```python
from build123d import *

# Parameters (mm, degrees)
F0_W           = 38.1
F0_H           = 6.35
F1_DEPTH       = 254
F3_D           = 9
F4_D           = 6
F4_CBORE_D     = 11
F4_CBORE_DEPTH = 3


with BuildPart() as f1:
    # F0 (on Top) → F1 (new body)
    with BuildSketch(Plane.XY):
        with Locations((19.05, 3.175)):
            Rectangle(F0_W, F0_H)
    extrude(amount=F1_DEPTH)

    # F3 (through all)
    with Locations(Plane.XZ):
        with Locations((19.05, 25.4), (19.05, 228.6)):
            Hole(F3_D / 2)

    # F4 (through all)
    with Locations(Plane.XZ):
        with Locations((19.05, 172.0088), (19.05, 81.9912)):
            CounterBoreHole(F4_D / 2, F4_CBORE_D / 2, F4_CBORE_DEPTH)


solid = f1.part
```
The listing builds one solid part. Answer for the finished solid, in the listing's coordinates (mm). A direction names the side the tool comes from. Coordinates: 2 decimals unless noted, no trailing zeros. Order: outer loops, then holes, each group sorted by start corner. A loop starts at its lowest first (then second) coordinate and runs counter-clockwise, first axis right, second up. Notation, with made-up numbers: M 38,34 L 87,34 A19 ccw 87,53 Z; hole C 19.5,-13 d10. An arc over 180 degrees is marked long. Answer as a JSON object with one key per item and string values. Group by question number.
1. Straight lines are drawn through the part: line 1 (Z direction, x = 19.05, y = 5); line 2 (Z direction, x = 19.05, y = 1.15); line 3 (X direction, y = 6.25, z = 82.5). For each, find the intervals that lie inside material, in ascending order.
2. A tool of negligible diameter and unlimited length cuts with its end or side. For faces 4 (the flat face through (21.4, 3, 169.6)), 5 (the cylindrical face through (20, 3, 233)), from which of +Z, -Z, +X, -X, +Y, -Y can it reach the whole face along a straight path? Write none if from no direction.
3. Section B-B on z = 228.6 is taken. Write down the section's boundary in (x, y).
4. Flat-ended cylindrical pins translate along their axes: P1, Ø10.5, axis at x = 19.05, z = 228.6, coming from the +Y side; P2, Ø7, axis at x = 19.05, z = 81.99, coming from the -Y side. Find the tip coordinate at first contact, or state that the pin passes through.
5. Section A-A on x = 19.05 is taken. Write down the section's boundary in (y, z), then the cut area to 3 significant figures.
6. Determine the mould class of faces 1 (the cylindrical face through (18.33, 1.48, 177.46)), 2 (the flat face through (0, 3, 125)), 3 (the flat face through (19, 0, 125)) for opening direction X: released by +X, released by -X, zero draft, split by the parting line, or undercut.
7. Section C-C on y = 2 is taken. Write down the section's boundary in (x, z).
Values follow:
{
 "1": {"line 1": "0 to 20.9, 29.9 to 78.99, 84.99 to 169.01, 175.01 to 224.1, 233.1 to 254", "line 2": "0 to 20.9, 29.9 to 76.49, 87.49 to 166.51, 177.51 to 224.1, 233.1 to 254", "line 3": "0 to 16.09, 22.01 to 38.1"},
 "2": {"face 4": "-Y", "face 5": "+Y, -Y"},
 "3": {"outline": "M 0,0 L 14.55,0 L 14.55,6.35 L 0,6.35 Z; M 23.55,0 L 38.1,0 L 38.1,6.35 L 23.55,6.35 Z"},
 "4": {"P1": "y = 6.35", "P2": "y = 3"},
 "5": {"outline": "M 0,0 L 6.35,0 L 6.35,20.9 L 0,20.9 Z; M 0,29.9 L 6.35,29.9 L 6.35,78.99 L 3,78.99 L 3,76.49 L 0,76.49 Z; M 0,87.49 L 3,87.49 L 3,84.99 L 6.35,84.99 L 6.35,169.01 L 3,169.01 L 3,166.51 L 0,166.51 Z; M 0,177.51 L 3,177.51 L 3,175.01 L 6.35,175.01 L 6.35,224.1 L 0,224.1 Z; M 0,233.1 L 6.35,233.1 L 6.35,254 L 0,254 Z", "area": "1,390 mm2"},
 "6": {"face 1": "undercut", "face 2": "released by -X", "face 3": "zero draft"},
 "7": {"outline": "M 0,0 L 38.1,0 L 38.1,254 L 0,254 Z; hole C 19.05,81.99 d11; hole C 19.05,172.01 d11; hole C 19.05,25.4 d9; hole C 19.05,228.6 d9"}
}
